from build123d import *

# Parameters (mm, degrees)
SKETCH_1_W          = 30
SKETCH_1_H          = 32
EXTRUDE_1_DEPTH     = 7
EXTRUDE_2_DEPTH     = 30
SKETCH_3_W          = 30
SKETCH_3_H          = 10
SKETCH_3_R          = 2.6
SKETCH_3_R_2        = 2.5
EXTRUDE_3_DEPTH     = 4
CUT_EXTRUDE_1_DEPTH = 60


with BuildPart() as part:
    # Эскиз1 → Бобышка-Вытянуть1 (new body)
    with BuildSketch(Plane.XY):
        with Locations((15, 16)):
            Rectangle(SKETCH_1_W, SKETCH_1_H)
    extrude(amount=EXTRUDE_1_DEPTH)

    # Эскиз2 → Бобышка-Вытянуть2 (add)
    with BuildSketch(Plane.ZY):
        with BuildLine():
            Line((7, 32), (17.940751301, 32))
            Line((17.940751301, 32), (17.940751301, 28.35))
            ThreePointArc((17.940751301, 28.35), (9, 16), (17.940751301, 3.65))
            Line((17.940751301, 3.65), (17.940751301, 0))
            Line((17.940751301, 0), (7, 0))
            Line((7, 0), (7, 32))
        make_face()
    extrude(amount=-EXTRUDE_2_DEPTH)

    # Эскиз3 → Бобышка-Вытянуть3 (add)
    # profile 1 of 2: a face of its own
    with BuildSketch(Plane(origin=(0, 0, 17.940751301), x_dir=(-1, 0, 0), z_dir=(0, 0, -1))):
        with Locations((-15, 37)):
            Rectangle(SKETCH_3_W, SKETCH_3_H)
        with Locations(Location((-25, 37, 0), (0, 0, 180))):
            Circle(SKETCH_3_R, mode=Mode.SUBTRACT)
        with Locations(Location((-5, 37, 0), (0, 0, 180))):
            Circle(SKETCH_3_R_2, mode=Mode.SUBTRACT)
    # profile 2 of 2: a face of its own
    with BuildSketch(Plane(origin=(0, 0, 17.940751301), x_dir=(-1, 0, 0), z_dir=(0, 0, -1))):
        with Locations((-15, -5)):
            Rectangle(SKETCH_3_W, SKETCH_3_H)
        with Locations(Location((-25, -5, 0), (0, 0, 180))):
            Circle(SKETCH_3_R_2, mode=Mode.SUBTRACT)
        with Locations(Location((-5, -5, 0), (0, 0, 180))):
            Circle(SKETCH_3_R, mode=Mode.SUBTRACT)
    extrude(amount=EXTRUDE_3_DEPTH)

    # Эскиз4 → Вырез-Вытянуть1 (cut)
    with BuildSketch(Plane(origin=(30, 0, 0), x_dir=(0, 0, -1), z_dir=(1, 0, 0))):
        with BuildLine():
            Line((-13.940751301, 32), (0, 32))
            Line((0, 32), (0, 0))
            Line((0, 0), (-13.940751301, 0))
            ThreePointArc((-13.940751301, 0), (-0.73723231, 16), (-13.940751301, 32))
        make_face()
    extrude(amount=-CUT_EXTRUDE_1_DEPTH, mode=Mode.SUBTRACT)


solid = part.part
Here's how the part is built. I have some questions about the finished solid (model axes, mm). A direction names the side the tool comes from. Coordinates: 2 decimals unless noted, no trailing zeros. Order: outer loops, then holes, each group sorted by start corner. A loop starts at its lowest first (then second) coordinate and runs counter-clockwise, first axis right, second up. Notation, with made-up numbers: (89.5, -39) -> (129.5, -39) arc R23 cw to (129.5, -21) -> close; hole circle Ø6 at (84.5, 27.25). An arc over 180 degrees is marked (long way). Answer in a Markdown table with one row per item.
(1) I want a section at A-A on x = 25. List the corners of the cut face in (y, z) for me, then the cut area to 3 significant figures.
Answer key:
| item | result |
|---|---|
| outline | (-10, 13.94) -> (-7.5, 13.94) -> (-7.5, 17.94) -> (-10, 17.94) -> close; (-2.5, 13.94) -> (0, 13.94) arc R16.3 ccw to (32, 13.94) -> (34.4, 13.94) -> (34.4, 17.94) -> (28.35, 17.94) arc R13 cw to (3.65, 17.94) -> (-2.5, 17.94) -> close; (39.6, 13.94) -> (42, 13.94) -> (42, 17.94) -> (39.6, 17.94) -> close |
| area | 322 mm^2 |
(2) Please list where these lines run through material, in increasing order: probe 1 along X at (y, z) = (37, 15.85); probe 2 along X at (y, z) = (-5, 15.65); probe 3 along Y at (x, z) = (5, 16.9).
Answer key:
| item | result |
|---|---|
| probe 1 | 0 to 2.5, 7.5 to 22.4, 27.6 to 30 |
| probe 2 | 0 to 2.4, 7.6 to 22.5, 27.5 to 30 |
| probe 3 | -10 to -7.6, -2.4 to 4.04, 27.96 to 34.5, 39.5 to 42 |
(3) Thinking about a two-plate mould opening in Y: for faces 4 (the face through (24.44, 39.54, 15.97)), 5 (the face through (15, 42, 16)), 6 (the face through (15, 35, 17.941)), which applies, +Y half, -Y half, draft (parallel to the pull), parting line (faces both ways), or undercut?
Answer key:
| item | result |
|---|---|
| face 4 | undercut |
| face 5 | +Y half |
| face 6 | draft |
(4) On a 3-axis mill with a long thin cutter (end or side, diameter ignored), from which of +Z, -Z, +X, -X, +Y, -Y can I reach the whole of each face in a straight line? I mean faces 1 (the face through (15, -5, 13.941)), 2 (the face through (7.385, 36.249, 15.969)), 3 (the face through (15, 37, 13.941)). Say none if no direction works.
Answer key:
| item | result |
|---|---|
| face 1 | -Z, +X, -X, -Y |
| face 2 | +Z, -Z |
| face 3 | -Z, +X, -X, +Y |
(5) I want a section at C-C on y = -5. List the corners of the cut face in (x, z) for me.
Answer key:
| item | result |
|---|---|
| outline | (0, 13.94) -> (2.4, 13.94) -> (2.4, 17.94) -> (0, 17.94) -> close; (7.6, 13.94) -> (22.5, 13.94) -> (22.5, 17.94) -> (7.6, 17.94) -> close; (27.5, 13.94) -> (30, 13.94) -> (30, 17.94) -> (27.5, 17.94) -> close |
(6) I want a section at D-D on z = 13.25. List the corners of the cut face in (x, y) for me.
Answer key:
| item | result |
|---|---|
| outline | (0, 0.15) -> (30, 0.15) -> (30, 6.39) -> (0, 6.39) -> close; (0, 25.61) -> (30, 25.61) -> (30, 31.85) -> (0, 31.85) -> close |
(7) I want a section at B-B on z = 16. List the corners of the cut face in (x, y) for me.
Answer key:
| item | result |
|---|---|
| outline | (0, -10) -> (30, -10) -> (30, 4.47) -> (0, 4.47) -> close; (0, 27.53) -> (30, 27.53) -> (30, 42) -> (0, 42) -> close; hole circle Ø5.2 at (5, -5); hole circle Ø5 at (5, 37); hole circle Ø5.2 at (25, 37); hole circle Ø5 at (25, -5) |
(8) Will these pins go through, and if not, where does the flat tip stop? pin 1 Ø8 at (x, y) = (13, -5.5) entering from -Z; pin 2 Ø8 at (x, z) = (15, 2.5) entering from -Y; pin 3 Ø4 at (y, z) = (23, 9) entering from -X; pin 4 Ø3 at (x, y) = (25, -5) entering from -Z.
Answer key:
| item | result |
|---|---|
| pin 1 | z = 13.94 |
| pin 2 | y = 3.57 |
| pin 3 | x = 0 |
| pin 4 | through |
